```python
from build123d import *

# Parameters (mm, degrees)
SKETCH1_R           = 20
BOSS_EXTRUDE1_DEPTH = 120
SKETCH2_R           = 25
CUT_EXTRUDE1_DEPTH  = 110
SKETCH3_R           = 10
BOSS_EXTRUDE2_DEPTH = 120


with BuildPart() as part:
    # Sketch1 → Boss-Extrude1 (new body)
    with BuildSketch(Plane.XY):
        with BuildLine():
            Line((0, 0), (-55, 0))
            ThreePointArc((-55, 0), (-90, 35), (-55, 70))
            Line((-55, 70), (0, 70))
            Line((0, 70), (0, 0))
        make_face()
        with Locations((-55, 35)):
            Circle(SKETCH1_R, mode=Mode.SUBTRACT)
    extrude(amount=BOSS_EXTRUDE1_DEPTH)

    # Sketch2 → Cut-Extrude1 (cut)
    with BuildSketch(Plane.XY.offset(120)):
        with Locations((-55, 35)):
            Circle(SKETCH2_R)
    extrude(amount=-CUT_EXTRUDE1_DEPTH, mode=Mode.SUBTRACT)

    # Sketch3 → Boss-Extrude2 (add)
    with BuildSketch(Plane(origin=(0, 0, 0), x_dir=(0, 0, -1), z_dir=(1, 0, 0))):
        with Locations(Location((-35, 35, 0), (0, 0, 180))):
            Circle(SKETCH3_R)
    extrude(amount=BOSS_EXTRUDE2_DEPTH)


solid = part.part
```
Work out the finished part from the listing and answer in its coordinate system (mm). A direction names the side the tool comes from. Round coordinates to 2 decimals unless told otherwise and drop trailing zeros. Write each loop counter-clockwise with the first axis right and the second up, starting at its lowest first coordinate (ties: lowest second). Pieces come first, ordered by that corner, then holes.
1) A cutting plane is placed at A-A on y = 35. Determine the outline of the cut face in (x, z).
2) A cutting plane is placed at D-D on z = 88.5. Determine the outline of the cut face in (x, y), and give its area (3 significant figures).
3) A cutting plane is placed at C-C on x = -48. Determine the outline of the cut face in (y, z) (3 decimals).
4) Consider probe 1 along X at (y, z) = (35, 6); probe 2 along Y at (x, z) = (-55, 46); probe 3 along Y at (x, z) = (-55, 3). Determine where each line is inside the solid, lowest interval first.
5) Which of the six approach directions +Z, -Z, +X, -X, +Y, -Y give full straight-line access (tool end or side, diameter ignored) to faces 1 (the face through (59.16, 44.76, 32.83)), 2 (the face through (-34, 35, 0)), 3 (the face through (-75, 20, 66))?
6) A cutting plane is placed at B-B on z = 35. Determine the outline of the cut face in (x, y).
7) Determine the mould class of faces 4 (the face through (-89.99, 34.23, 59.16)), 5 (the face through (-35.924, 41.007, 4.93)), 6 (the face through (-24, 35, 120)) for opening direction X: pulls with the +X half, pulls with the -X half, needs draft (parallel to the pull), parting line crosses it, or undercut.
8) Flat-ended cylindrical pins translate along their axes: P1, Ø21, axis at y = 26, z = 65.5, coming from the +X side; P2, Ø25, axis at x = -48, y = 28, coming from the +Z side; P3, Ø3, axis at y = 19.5, z = 24, coming from the -X side. Find the tip coordinate at first contact, or state that the pin passes through.
Entries:
1. outline: (-90, 0) - (-75, 0) - (-75, 10) - (-80, 10) - (-80, 120) - (-90, 120) - close; (-35, 0) - (0, 0) - (0, 25) - (120, 25) - (120, 45) - (0, 45) - (0, 120) - (-30, 120) - (-30, 10) - (-35, 10) - close
2. outline: (-55, 0) - (0, 0) - (0, 70) - (-55, 70) arc R35 ccw to start; hole circle Ø50 at (-55, 35)
2. area: 3,810 mm2
3. outline: (0, 0) - (16.265, 0) - (16.265, 10) - (11, 10) - (11, 120) - (0, 120) - close; (53.735, 0) - (70, 0) - (70, 120) - (59, 120) - (59, 10) - (53.735, 10) - close
4. probe 1: x = -90 to -75, -35 to 0
4. probe 2: y = 0 to 10, 60 to 70
4. probe 3: y = 0 to 15, 55 to 70
5. face 1: +X
5. face 2: -Z, +X, -X, +Y, -Y
5. face 3: +Z
6. outline: (-55, 0) - (0, 0) - (0, 25) - (120, 25) - (120, 45) - (0, 45) - (0, 70) - (-55, 70) arc R35 ccw to start; hole circle Ø50 at (-55, 35)
7. face 4: pulls with the -X half
7. face 5: undercut
7. face 6: needs draft
8. P1: stops at x = 0
8. P2: stops at z = 10
8. P3: stops at x = -87.08
